The drawing under review shows one solid part. Ordinate dimensions are in mm from its lowest x, y, z. A direction names the side the tool comes from. Round coordinates to 2 decimals unless told otherwise and drop trailing zeros. Write each loop counter-clockwise with the first axis right and the second up, starting at its lowest first coordinate (ties: lowest second). Pieces come first, ordered by that corner, then holes. Notation, with made-up numbers: (-19, -36) -> (29, -36) arc R14 ccw to (29, -20) -> close; hole circle Ø5 at (-14, 28). An arc over 180 degrees is marked (long way). Write item = value, one per line. Start each with the question number.
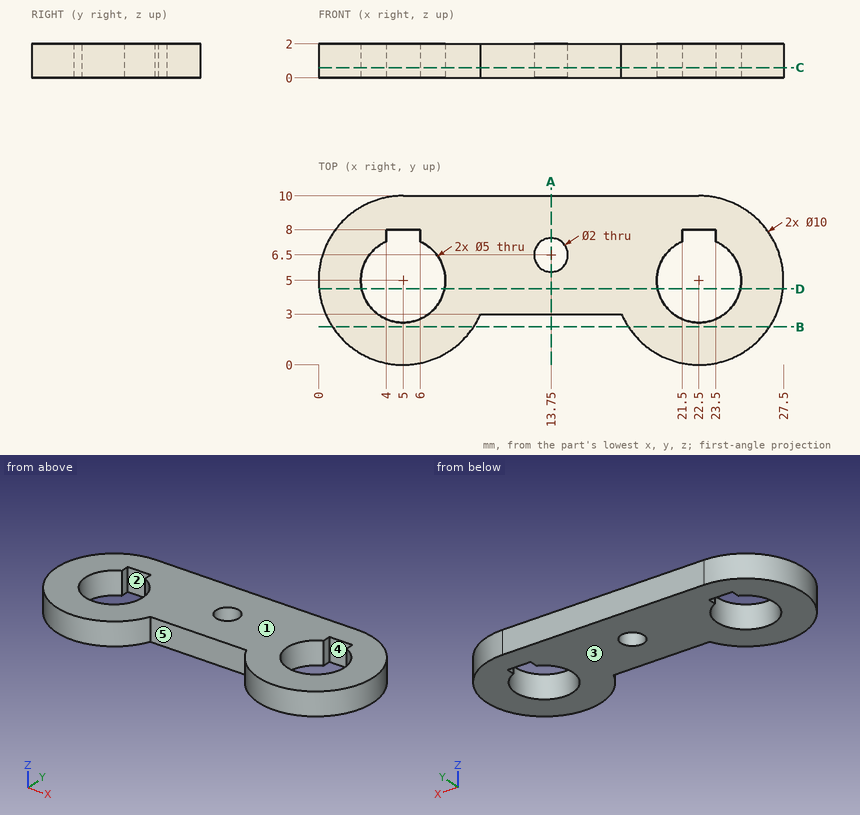
1. Consider section A-A, the plane x = 13.75. Give the boundary of the cut face in (y, z), then the cut area to 3 significant figures.
2. Clearance check with flat-ended pins moving along their axes: pin 1 Ø0.8 at (y, z) = (8, 0.5) entering from -X; pin 2 Ø6 at (x, y) = (22.5, 5) entering from +Z; pin 3 Ø1 at (x, z) = (12.5, 1.5) entering from -Y. State where each tip first meets the part, or that it passes through.
3. Draft analysis for pull direction X (two halves, no side actions). For the marked faces 1 and 2, state which applies: +X half, -X half, draft (parallel to the pull), parting line (faces both ways), or undercut.
4. Machinability: for the marked faces 3, 4 and 5, which of the approach directions +Z, -Z, +X, -X, +Y, -Y give a long, thin tool a straight path to every point of the face, cutting with its end or side? Answer none if there is none.
5. Wall thickness on L1, parallel to X at y = 5, z = 0.65; L2, parallel to Y at x = 22.5, z = 1.3; L3, parallel to X at y = 4, z = 1.6: over which ranges is each line inside the solid? List them lowest first. Write a range as from..to.
6. Consider section D-D, the plane y = 4.5. Give the boundary of the cut face in (x, z), then the cut area to 3 significant figures.
7. Consider section B-B, the plane y = 2.25. Give the boundary of the cut face in (x, z).
8. Consider section C-C, the plane z = 0.6. Give the boundary of the cut face in (x, y).
Outcome:
q1.outline = (3, 0) -> (5.5, 0) -> (5.5, 2) -> (3, 2) -> close; (7.5, 0) -> (10, 0) -> (10, 2) -> (7.5, 2) -> close
q1.area = 10.0 mm2
q2.pin_1 = 0.73
q2.pin_2 = 2
q2.pin_3 = 3
q3.face_1 = draft
q3.face_2 = undercut
q4.face_3 = -Z, +X, -X, +Y, -Y
q4.face_4 = +Z, -Z
q4.face_5 = +Z, -Z, -Y
q5.L1 = 0..2.5, 7.5..20, 25..27.5
q5.L2 = 0..2.5, 8..10
q5.L3 = 0.1..2.71, 7.29..20.21, 24.79..27.4
q6.outline = (0.03, 0) -> (2.55, 0) -> (2.55, 2) -> (0.03, 2) -> close; (7.45, 0) -> (20.05, 0) -> (20.05, 2) -> (7.45, 2) -> close; (24.95, 0) -> (27.47, 0) -> (27.47, 2) -> (24.95, 2) -> close
q6.area = 35.3 mm2
q7.outline = (0.82, 0) -> (9.18, 0) -> (9.18, 2) -> (0.82, 2) -> close; (18.32, 0) -> (26.68, 0) -> (26.68, 2) -> (18.32, 2) -> close
q8.outline = (5, 10) arc R5 ccw (long way) to (9.58, 3) -> (17.92, 3) arc R5 ccw (long way) to (22.5, 10) -> close; hole (4, 7.29) arc R2.5 ccw (long way) to (6, 7.29) -> (6, 8) -> (4, 8) -> close; hole circle Ø2 at (13.75, 6.5); hole (21.5, 7.29) arc R2.5 ccw (long way) to (23.5, 7.29) -> (23.5, 8) -> (21.5, 8) -> close
